Autodesk Inventor part; units mm, degrees
ref_plane "YZ Plane" through (0, 0, 0) normal (1, 0, 0) x (0, 1, 0)
ref_plane "XZ Plane" through (0, 0, 0) normal (0, 1, 0) x (-1, 0, 0)
ref_plane "XY Plane" through (0, 0, 0) normal (0, 0, 1) x (1, 0, 0)
sketch "Sketch1" plane through (0, 0, 0) normal (0, 1, 0) x (-1, 0, 0)
  line L0 (-0.3716, 0) -> (46.6284, 0) construction
  line L1 (46.6284, 0) -> (46.6284, -99) construction
  line L2 (46.6284, -100) -> (-0.3716, -100) construction
  line L3 (-0.3716, -100) -> (-0.3716, -1) construction
  circle A0 centre (3.6284, -4) radius 1.6 construction
  circle A1 centre (42.6284, -4) radius 1.6 construction
  circle A2 centre (42.6284, -96) radius 1.729 construction
  line L4 (23.1284, 0) -> (23.1284, -100) construction
  line L5 (23.1284, -13) -> (18.1284, -13) construction
  line L6 (18.1284, -13) -> (0.1284, -13) construction
  line L7 (23.1284, -13) -> (46.1284, -13) construction
  line L8 (45.6284, -10.5) -> (45.6284, -89.5)
  line L9 (10.1284, -1) -> (36.1284, -1)
  line L10 (0.6284, -99) -> (36.1284, -99)
  line L11 (0.6284, -10.5) -> (0.6284, -99)
  line L12 (36.9206, -1) -> (49.2353, -1) construction
  line L13 (45.6284, -1) -> (36.1284, -1) construction
  line L14 (36.1284, -1) -> (45.6284, -10.5)
  line L15 (36.1284, -99) -> (45.6284, -89.5)
  line L16 (36.1284, -99) -> (49.5635, -99) construction
  line L17 (0.6284, -1) -> (10.1284, -1) construction
  line L18 (10.1284, -1) -> (0.6284, -10.5)
  circle A3 centre (3.6284, -4) radius 1.6
  circle A4 centre (42.6284, -4) radius 1.6
  circle A5 centre (42.6284, -96) radius 1.729
  circle A6 centre (61, -38.5) radius 1.6
  circle A7 centre (61, -50.5) radius 1.6
  line L19 (47.6284, -34.5) -> (64, -34.5)
  line L20 (64, -34.5) -> (64, -54.5)
  line L21 (64, -54.5) -> (47.6284, -54.5)
  circle A8 centre (-14, -38.5) radius 1.6
  circle A9 centre (-14, -50.5) radius 1.6
  line L22 (-1.3716, -34.5) -> (-17, -34.5)
  line L23 (-17, -34.5) -> (-17, -54.5)
  line L24 (-17, -54.5) -> (-1.3716, -54.5)
  line L25 (47.6284, -101) -> (47.6284, -54.5)
  line L26 (47.6284, -34.5) -> (47.6284, 1)
  line L27 (-1.3716, -101) -> (-1.3716, -54.5)
  line L28 (-1.3716, -34.5) -> (-1.3716, 1)
  line L29 (47.6284, 1) -> (-1.3716, 1)
  line L30 (47.6284, -101) -> (-1.3716, -101)
  dimension "d0" = 47
  dimension "d1" = 100
  dimension "d2" = 3.2
  dimension "d3" = 4
  dimension "d4" = 4
  dimension "d5" = 4
  dimension "d6" = 43
  dimension "d7" = 3.2
  dimension "d8" = 43
  dimension "d9" = 96
  dimension "d10" = 23.5
  dimension "d11" = 5
  dimension "d12" = 13
  dimension "d13" = 18
  dimension "d15" = 23
  dimension "d24" = 1
  dimension "d33" = 8.7079
  dimension "d34" = 9.5
  dimension "d35" = 45
  dimension "d36" = 45
  dimension "d37" = 9.5
  dimension "d38" = 45
  dimension "d39" = 3.2
  dimension "d42" = 3.2
  dimension "d43" = 12
  dimension "d44" = 4
  dimension "d45" = 3
  dimension "d46" = 4
  dimension "d47" = 3.2
  dimension "d49" = 3.2
  dimension "d50" = 12
  dimension "d51" = 3
extrude "Extrusion1" add sketch "Sketch1" along normal blind 2
fillet "Fillet1" radius 2 18 edges at (-45.6284, 1, -89.5) (-36.1284, 1, -99) (-64, 1, -34.5) (-47.6284, 1, 1) (1.3716, 1, 1) (17, 1, -34.5) (1.3716, 1, -34.5) (17, 1, -54.5) (1.3716, 1, -54.5) (1.3716, 1, -101) (-47.6284, 1, -101) (-64, 1, -54.5) (-45.6284, 1, -10.5) (-36.1284, 1, -1) (-10.1284, 1, -1) (-0.6284, 1, -10.5) (-47.6284, 1, -54.5) (-0.6284, 1, -99)
properties part number "PCB Holder"
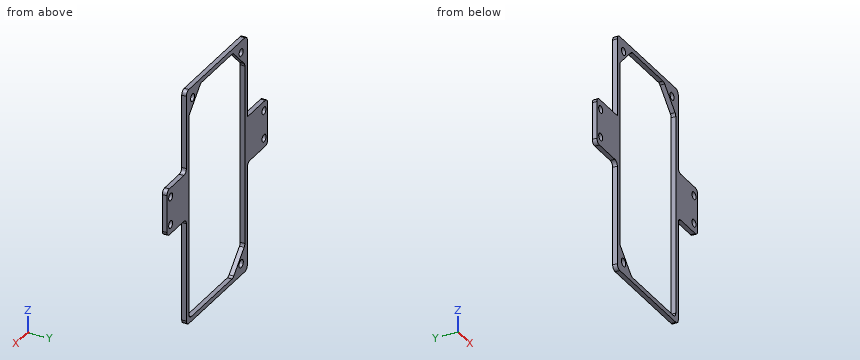
Verification items for the finished model (mm, model axes). Coordinates: 2 decimals unless noted, no trailing zeros. Loops run counter-clockwise (first coordinate to the right, second up) from the corner with the lowest first, then second, coordinate; pieces in that order, holes last. Notation, with made-up numbers: (27, 12.5) -> (55, 12.5) arc R26 ccw to (55, 47.5) -> close; hole circle Ø10 at (76, 13). An arc over 180 degrees is marked (long way). Answer as a JSON object with one key per item and string values. Group by question number.
Item 1: Sectioned sample at B-B on x = -29.5. Record the boundary of the cut face in (y, z), plus the area to 3 significant figures.
Item 2: Sectioned sample at C-C on z = -22.5. Record the boundary of the cut face in (x, y).
Item 3: Depth check by flat-ended pin: pin 1 (0.6 mm diameter, centred on x = 7.5, y = 0.5, fed in from -Z); pin 2 (4 mm diameter, centred on x = 14, z = -50.5, fed in from -Y); pin 3 (1 mm diameter, centred on y = 1, z = -20, fed in from -X); pin 4 (1 mm diameter, centred on y = 0.5, z = -9.5, fed in from +X). Enter the tip coordinate at first touch or a pass-through.
Item 4: Sectioned sample at A-A on z = -38.5. Record the boundary of the cut face in (x, y), plus the area to 3 significant figures.
Item 5: Scan lines: probe 1 along Z at (x, y) = (14, 1.15); probe 2 along Z at (x, y) = (-28, 1.65); probe 3 along X at (y, z) = (1.1, -96). Record each from-to range of solid material in increasing order.
Item 6: Sectioned sample at D-D on x = -43. Record the boundary of the cut face in (y, z).
Evaluation:
{
 "1": {"outline": "(0, -101) -> (2, -101) -> (2, -99) -> (0, -99) -> close; (0, -1) -> (2, -1) -> (2, 1) -> (0, 1) -> close", "area": "8.00 mm²"},
 "2": {"outline": "(-47.63, 0) -> (-45.63, 0) -> (-45.63, 2) -> (-47.63, 2) -> close; (-0.63, 0) -> (1.37, 0) -> (1.37, 2) -> (-0.63, 2) -> close"},
 "3": {"pin 1": "stops at z = -54.5", "pin 2": "stops at y = 0", "pin 3": "stops at x = -47.63", "pin 4": "stops at x = 1.37"},
 "4": {"outline": "(-64, 0) -> (-62.6, 0) -> (-62.6, 2) -> (-64, 2) -> close; (-59.4, 0) -> (-45.63, 0) -> (-45.63, 2) -> (-59.4, 2) -> close; (-0.63, 0) -> (12.4, 0) -> (12.4, 2) -> (-0.63, 2) -> close; (15.6, 0) -> (17, 0) -> (17, 2) -> (15.6, 2) -> close", "area": "59.2 mm²"},
 "5": {"probe 1": "z = -54.5 to -52.1, -48.9 to -40.1, -36.9 to -34.5", "probe 2": "z = -101 to -99, -1 to 1", "probe 3": "x = -47.63 to -44.36, -40.9 to -39.13, -0.63 to 1.37"},
 "6": {"outline": "(0, -101) -> (2, -101) -> (2, -97.69) -> (0, -97.69) -> close; (0, -94.31) -> (2, -94.31) -> (2, -92.13) -> (0, -92.13) -> close; (0, -7.87) -> (2, -7.87) -> (2, -5.56) -> (0, -5.56) -> close; (0, -2.44) -> (2, -2.44) -> (2, 1) -> (0, 1) -> close"}
}
